Geometry check sheet. Reference: the model listing, model coordinates, mm. A direction names the side the tool comes from. Give positions to 0.01 mm unless a question says otherwise; leave off trailing zeros. Write each loop counter-clockwise with the first axis right and the second up, starting at its lowest first coordinate (ties: lowest second). Pieces come first, ordered by that corner, then holes.
(1) Cross-section at D-D (x = 41). Record the boundary of the cut face in (y, z), and give its area (3 significant figures).
(2) Cross-section at A-A (z = -84). Record the boundary of the cut face in (x, y).
(3) Cross-section at C-C (y = 0.7). Count the separate pieces of the cut face and the enclosed holes in it, and give its area (3 significant figures).
(4) Mould release check, pull along X, two halves, no side actions. Record for faces 3 (the flat face through (49, 2, -73)), 4 (the flat face through (56.14, 0.99, -18.65)): +X half, -X half, draft (parallel to the pull), parting line (faces both ways), or undercut.
(5) Cross-section at B-B (x = 87). Record the boundary of the cut face in (y, z) (3 decimals), and give its area (3 significant figures).
(6) Tool access check on faces 1 (the flat face through (49, 0, -73)), 2 (the flat face through (79.723, 0.986, -58.508)). Record the directions out of +Z, -Z, +X, -X, +Y, -Y that give a thin tool (end or side, any length) a straight path to the whole face; none if there is none.
(7) Thickness scan on line 1 along Z through (x, y) = (12, 0.3); line 2 along X through (y, z) = (0.45, -21.5); line 3 along X through (y, z) = (0.4, -47). Record the ranges inside material, lowest first.
```python
from build123d import *

# Parameters (mm, degrees)
SKETCH1_W           = 100
SKETCH1_H           = 100
BOSS_EXTRUDE1_DEPTH = 2
FILLET1_R           = 1
FILLET2_R           = 1
CUT_EXTRUDE1_DEPTH  = 142.435497666


with BuildPart() as part:
    # Sketch1 → Boss-Extrude1 (new body)
    with BuildSketch(Plane(origin=(0, 0, 0), x_dir=(1, 0, 0), z_dir=(0, 1, 0))):
        with Locations((50, 50)):
            Rectangle(SKETCH1_W, SKETCH1_H)
        Polygon((10, 67.5), (30, 50), (10, 32.5), (10, 50), align=None, mode=Mode.SUBTRACT)
        Polygon((50, 30), (67.320508076, 40), (67.320508076, 60), (50, 70), (32.679491924, 60), (32.679491924, 40), align=None, mode=Mode.SUBTRACT)
        Polygon((90, 50), (90, 67.5), (70, 50), (90, 32.5), align=None, mode=Mode.SUBTRACT)
        Polygon((50, 10), (62.5, 10), (50, 27), (37.5, 10), align=None, mode=Mode.SUBTRACT)
        Polygon((50, 90), (62.5, 90), (50, 73), (37.5, 90), align=None, mode=Mode.SUBTRACT)
    extrude(amount=BOSS_EXTRUDE1_DEPTH)

    # Fillet1
    fillet1_edges = [part.edges().sort_by_distance(p)[0] for p in [
        (32.679491924, 1, -40),
        (50, 1, -30),
        (67.320508076, 1, -40),
        (67.320508076, 1, -60),
        (50, 1, -70),
        (32.679491924, 1, -60),
    ]]
    fillet(fillet1_edges, radius=FILLET1_R)

    # Fillet2
    fillet2_edges = [part.edges().sort_by_distance(p)[0] for p in [
        (90, 1, -32.5),
        (90, 1, -67.5),
        (70, 1, -50),
        (10, 1, -67.5),
        (10, 1, -32.5),
        (30, 1, -50),
        (37.5, 1, -10),
        (62.5, 1, -10),
        (50, 1, -27),
        (37.5, 1, -90),
        (50, 1, -73),
        (62.5, 1, -90),
    ]]
    fillet(fillet2_edges, radius=FILLET2_R)

    # Sketch2 → Cut-Extrude1 (cut, through all)
    with BuildSketch(Plane(origin=(0, 2, 0), x_dir=(1, 0, 0), z_dir=(0, 1, 0))):
        with BuildLine():
            Line((11, 91), (11, 80))
            ThreePointArc((11, 80), (13, 78), (15, 80))
            Line((15, 80), (15, 91))
            ThreePointArc((15, 91), (13, 93), (11, 91))
        make_face()
        with BuildLine():
            Line((25, 91), (25, 80))
            ThreePointArc((25, 80), (27, 78), (29, 80))
            Line((29, 80), (29, 91))
            ThreePointArc((29, 91), (27, 93), (25, 91))
        make_face()
        with BuildLine():
            ThreePointArc((75, 80), (73, 78), (71, 80))
            Line((71, 80), (71, 91))
            ThreePointArc((71, 91), (73, 93), (75, 91))
            Line((75, 91), (75, 80))
        make_face()
        with BuildLine():
            ThreePointArc((89, 80), (87, 78), (85, 80))
            Line((85, 80), (85, 91))
            ThreePointArc((85, 91), (87, 93), (89, 91))
            Line((89, 91), (89, 80))
        make_face()
        with BuildLine():
            Line((89, 9), (89, 20))
            ThreePointArc((89, 20), (87, 22), (85, 20))
            Line((85, 20), (85, 9))
            ThreePointArc((85, 9), (87, 7), (89, 9))
        make_face()
        with BuildLine():
            Line((75, 9), (75, 20))
            ThreePointArc((75, 20), (73, 22), (71, 20))
            Line((71, 20), (71, 9))
            ThreePointArc((71, 9), (73, 7), (75, 9))
        make_face()
        with BuildLine():
            ThreePointArc((25, 20), (27, 22), (29, 20))
            Line((29, 20), (29, 9))
            ThreePointArc((29, 9), (27, 7), (25, 9))
            Line((25, 9), (25, 20))
        make_face()
        with BuildLine():
            ThreePointArc((11, 20), (13, 22), (15, 20))
            Line((15, 20), (15, 9))
            ThreePointArc((15, 9), (13, 7), (11, 9))
            Line((11, 9), (11, 20))
        make_face()
    extrude(amount=-CUT_EXTRUDE1_DEPTH, mode=Mode.SUBTRACT)


solid = part.part
```
Reply:
1. outline: (0, -100) - (2, -100) - (2, -90) - (0, -90) - close; (0, -85.24) - (2, -85.24) - (2, -64.8) - (0, -64.8) - close; (0, -35.2) - (2, -35.2) - (2, -14.76) - (0, -14.76) - close; (0, -10) - (2, -10) - (2, 0) - (0, 0) - close
1. area: 122 mm2
2. outline: (0, 0) - (11, 0) - (11, 2) - (0, 2) - close; (15, 0) - (25, 0) - (25, 2) - (15, 2) - close; (29, 0) - (41.91, 0) - (41.91, 2) - (29, 2) - close; (58.09, 0) - (71, 0) - (71, 2) - (58.09, 2) - close; (75, 0) - (85, 0) - (85, 2) - (75, 2) - close; (89, 0) - (100, 0) - (100, 2) - (89, 2) - close
3. separate pieces: 1
3. enclosed holes: 13
3. area: 7,390 mm2
4. face 3: draft
4. face 4: undercut
5. outline: (0, -100) - (2, -100) - (2, -93) - (0, -93) - close; (0, -78) - (2, -78) - (2, -64.875) - (0, -64.875) - close; (0, -35.125) - (2, -35.125) - (2, -22) - (0, -22) - close; (0, -7) - (2, -7) - (2, 0) - (0, 0) - close
5. area: 80.5 mm2
6. face 1: +Z, -Z, +X, -X, -Y
6. face 2: +Y, -Y
7. line 1: z = -100 to -92.73, -78.27 to -65.75, -34.25 to -21.73, -7.27 to 0
7. line 2: x = 0 to 11.68, 14.32 to 25.68, 28.32 to 45.96, 54.04 to 71.68, 74.32 to 85.68, 88.32 to 100
7. line 3: x = 0 to 10, 26.57 to 32.68, 67.32 to 73.43, 90 to 100
